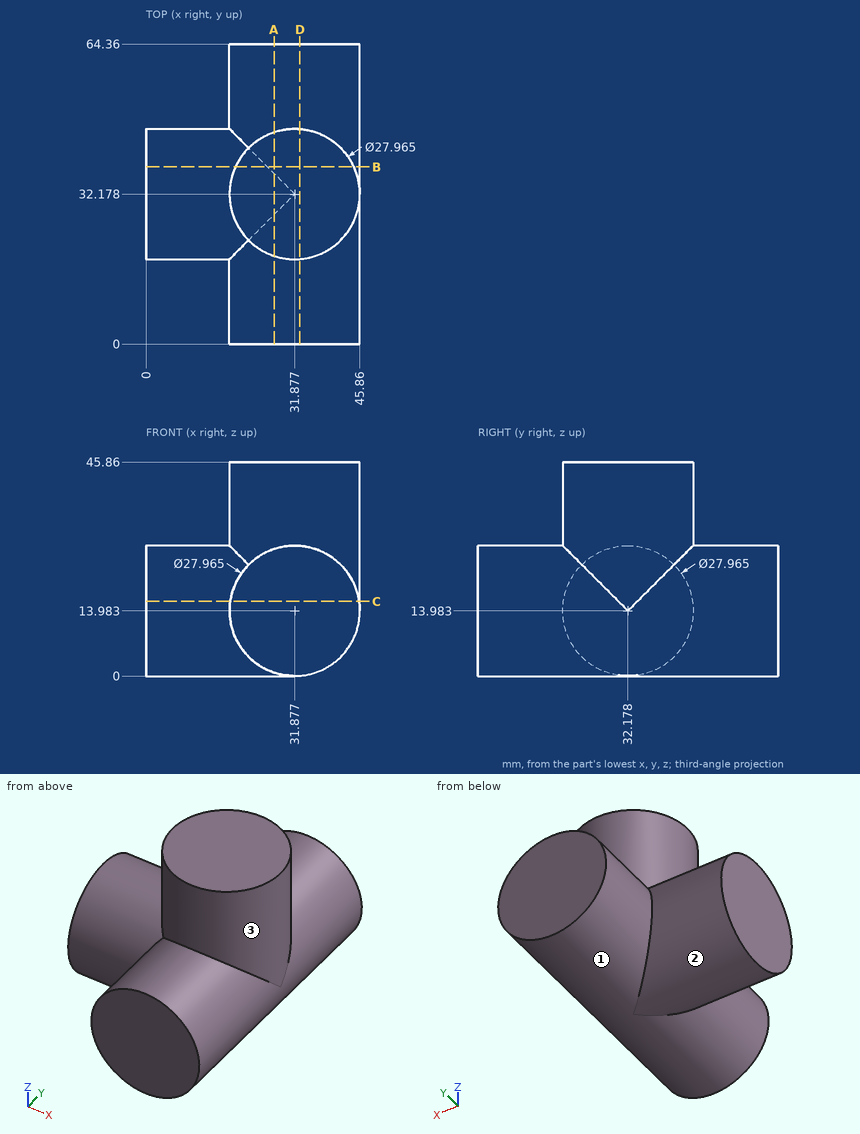
Geometry: see drawing. Coordinates: mm, zero at the bounding-box minimum. A direction names the side the tool comes from. Round coordinates to 2 decimals unless told otherwise and drop trailing zeros. Loops run counter-clockwise (first coordinate to the right, second up) from the corner with the lowest first, then second, coordinate; pieces in that order, holes last. Notation, with made-up numbers: M 50.5,22 L 104.5,22 A9 ccw 104.5,28 Z; hole C 44,85 d6. An arc over 180 degrees is marked long. Use a Markdown table: item, result. Add a question column.
1. Contact query for flat-ended pins moving along their axis: pin 1 (3 mm diameter, centred on y = 18, z = 37, fed in from -X); pin 2 (12 mm diameter, centred on y = 19, z = 30, fed in from -X); pin 3 (6 mm diameter, centred on y = 15.5, z = 25, fed in from -X); pin 4 (4 mm diameter, centred on y = 23, z = 16, fed in from -X). Output: stop coordinate, or through.
2. Ray query, line 1 along X through (y, z) = (33, 14.5); line 2 along X through (y, z) = (15, 16); line 3 along Y through (x, z) = (7.5, 7) (1 decimal). Return the intervals inside material, ascending. Write a range as [from, to].
3. Cut plane B-B, the plane y = 38. Output: boundary loops of the cut face in (x, z) (1 decimal).
4. Cut plane D-D, the plane x = 33. Output: boundary loops of the cut face in (y, z) (1 decimal).
5. Set-up query: the marked faces 1, 2 and 3. Return all of +Z, -Z, +X, -X, +Y, -Y with unobstructed straight access to the full face (end or side cutting, diameter ignored); none if empty.
6. Cut plane A-A, the plane x = 27.5. Output: boundary loops of the cut face in (y, z) (1 decimal).
7. Cut plane C-C, the plane z = 16. Output: boundary loops of the cut face in (x, y) (1 decimal), and give its area (3 significant figures).
Solution:
| question | item | result |
|---|---|---|
| 1 | pin 1 | stops at x = 25.98 |
| 1 | pin 2 | stops at x = 19.88 |
| 1 | pin 3 | stops at x = 20.42 |
| 1 | pin 4 | stops at x = 0 |
| 2 | line 1 | x = [0, 45.85] |
| 2 | line 2 | x = [18.04, 45.71] |
| 2 | line 3 | y = [20.1, 44.3] |
| 3 | outline | M 0,1.3 L 26.1,1.3 A14 ccw 44.6,19.8 L 44.6,45.9 L 19.2,45.9 L 19.2,26.7 L 0,26.7 Z |
| 4 | outline | M 0,0 L 64.4,0 L 64.4,27.9 L 46.1,27.9 L 46.1,45.9 L 18.2,45.9 L 18.2,27.9 L 0,27.9 Z |
| 5 | face 1 | none |
| 5 | face 2 | -X |
| 5 | face 3 | +Z |
| 6 | outline | M 0,0.7 L 27.8,0.7 A14 ccw 36.6,0.7 L 64.4,0.7 L 64.4,27.3 L 45.5,27.3 L 45.5,45.9 L 18.9,45.9 L 18.9,27.3 L 0,27.3 Z |
| 7 | outline | M 0,18.3 L 18,18.3 L 18,0 L 45.7,0 L 45.7,30.2 A14 ccw 45.7,34.2 L 45.7,64.4 L 18,64.4 L 18,46 L 0,46 Z |
| 7 | area | 2,280 mm2 |
